Can you work these out from the model? Positions are in its coordinate system, mm. A direction names the side the tool comes from. Give positions to 0.01 mm unless a question says otherwise; leave off trailing zeros. Loops run counter-clockwise (first coordinate to the right, second up) from the corner with the lowest first, then second, coordinate; pieces in that order, holes last. Notation, with made-up numbers: (18.25, 23.25) -> (77.25, 23.25) arc R13 cw to (77.25, 40.25) -> close; hole circle Ø6 at (22.25, 59.25). An arc over 180 degrees is marked (long way). Return JSON: item names as keys, results as strings. Group by question number.
Q1. Suppose I cut it at C-C, the plane z = 66. Please give me the cut outline in (x, y).
Q2. Will these pins go through, and if not, where does the flat tip stop? pin 1 (10 mm diameter, centred on y = -4, z = 72, fed in from -X); pin 2 (4 mm diameter, centred on x = 1.5, y = -6.5, fed in from +Z); pin 3 (2.5 mm diameter, centred on x = 3, z = 104, fed in from -Y).
Q3. Suppose I cut it at B-B, the plane x = 0. Please give me the cut outline in (y, z).
Q4. Suppose I cut it at A-A, the plane y = 0. Please give me the cut outline in (x, z).
Q5. I need wall thicknesses on line 1 along Z through (x, y) = (6.5, 4.5); line 2 along X through (y, z) = (-3, 73); line 3 along Z through (x, y) = (-4, -0.75). Which ranges of each line are inside material? Lowest first, please. Write a range as [from, to].
Q6. Suppose I cut it at D-D, the plane y = 7.25. Please give me the cut outline in (x, z).
Q7. Which directions (+Z, -Z, +X, -X, +Y, -Y) give clear straight access to the entire face, cutting with the end or side of a thin tool? Please do faces 4 (the cylindrical face through (4.57, 7.167, 1.972)), 5 (the flat face through (1, 0, 104)), 6 (the cylindrical face through (-3.905, -0.867, 102.535)).
Q8. Thinking about a two-plate mould opening in Y: for faces 1 (the flat face through (2, -1, 104)), 2 (the flat face through (0, 0, 105)), 3 (the cylindrical face through (-1.08, -4.88, 51.33)), which applies, pulls with the +Y half, pulls with the -Y half, needs draft (parallel to the pull), parting line crosses it, or undercut?
```python
from build123d import *

# Parameters (mm, degrees)
F0_R     = 8.5
F1_DEPTH = 4
F3_R     = 5
F4_DEPTH = 100
F5_W     = 4
F5_H     = 5
F9_DEPTH = 3


with BuildPart() as f1:
    # F0 (on Top) → F1 (new body)
    with BuildSketch(Plane.XY):
        Circle(F0_R)
    extrude(amount=F1_DEPTH)

    # F3 (on Top) → F4 (join)
    with BuildSketch(Plane.XY):
        Circle(F3_R)
    extrude(amount=F4_DEPTH)

    # F5 (on Right) → F6 (revolve)
    with BuildSketch(Plane.YZ):
        with Locations((2, 102.5)):
            Rectangle(F5_W, F5_H)
    revolve(axis=Axis((0, 0, 102.5), (0, 0, -1)))

    # F8 (on face) → F9 (cut)
    with BuildSketch(Plane.XY.offset(105)):
        with BuildLine():
            Line((3.8729833462, 1), (1, 1))
            Line((1, 1), (1, -1))
            Line((1, -1), (3.8729833462, -1))
            ThreePointArc((3.8729833462, -1), (3.9681187851, -0.5040171699), (4, 0))
            ThreePointArc((4, 0), (3.9681187851, 0.5040171699), (3.8729833462, 1))
        make_face()
    extrude(amount=-F9_DEPTH, mode=Mode.SUBTRACT)


solid = f1.part
```
Ans:
{
 "1": {"outline": "circle Ø10 at (0, 0)"},
 "2": {"pin 1": "stops at x = -5", "pin 2": "stops at z = 100", "pin 3": "stops at y = -3.6"},
 "3": {"outline": "(-8.5, 0) -> (8.5, 0) -> (8.5, 4) -> (5, 4) -> (5, 100) -> (4, 100) -> (4, 105) -> (-4, 105) -> (-4, 100) -> (-5, 100) -> (-5, 4) -> (-8.5, 4) -> close"},
 "4": {"outline": "(-8.5, 0) -> (8.5, 0) -> (8.5, 4) -> (5, 4) -> (5, 100) -> (4, 100) -> (4, 102) -> (1, 102) -> (1, 105) -> (-4, 105) -> (-4, 100) -> (-5, 100) -> (-5, 4) -> (-8.5, 4) -> close"},
 "5": {"line 1": "z = [0, 4]", "line 2": "x = [-4, 4]", "line 3": "z = [0, 100]"},
 "6": {"outline": "(-4.44, 0) -> (4.44, 0) -> (4.44, 4) -> (-4.44, 4) -> close"},
 "7": {"face 4": "+Z, -Z", "face 5": "+Z, +X", "face 6": "+Z"},
 "8": {"face 1": "undercut", "face 2": "needs draft", "face 3": "parting line crosses it"}
}
